Here's how the part is built. I have some questions about the finished solid (model axes, mm). A direction names the side the tool comes from. Round coordinates to 2 decimals unless told otherwise and drop trailing zeros. Loops run counter-clockwise (first coordinate to the right, second up) from the corner with the lowest first, then second, coordinate; pieces in that order, holes last. Notation, with made-up numbers: (-4.75, 68) -> (51.25, 68) arc R21 ccw to (51.25, 76) -> close; hole circle Ø4 at (8, -37). An arc over 180 degrees is marked (long way). Use CSV: the item, a comma, the result in double quotes. Start each with the question number.
from build123d import *

# Parameters (mm, degrees)
F1_DEPTH = 910
F3_DEPTH = 125.001
F5_DEPTH = 65.001
F6_R     = 9
F7_DEPTH = 7.5
F8_R     = 9
F9_DEPTH = 7.5


with BuildPart() as f1:
    # F0 (on Front) → F1 (new body)
    with BuildSketch(Plane.XZ):
        with BuildLine():
            Line((0, 125), (0, 0))
            Line((0, 0), (65, 0))
            Line((65, 0), (65, 7.5))
            Line((65, 7.5), (12.7, 7.5))
            ThreePointArc((12.7, 7.5), (7.043146, 9.843146), (4.7, 15.5))
            Line((4.7, 15.5), (4.7, 109.5))
            ThreePointArc((4.7, 109.5), (7.043146, 115.156854), (12.7, 117.5))
            Line((12.7, 117.5), (65, 117.5))
            Line((65, 117.5), (65, 125))
            Line((65, 125), (0, 125))
        make_face()
    extrude(amount=F1_DEPTH)

    # F2 (on face) → F3 (cut, through all)
    with BuildSketch(Plane.XY.offset(125)):
        Polygon((65, -65), (65, 0), (0, 0), align=None)
    extrude(amount=-F3_DEPTH, mode=Mode.SUBTRACT)

    # F4 (on face) → F5 (cut, through all)
    with BuildSketch(Plane(origin=(0, 0, 0), x_dir=(0, -1, 0), z_dir=(-1, 0, 0))):
        Polygon((910, 0), (910, 125), (785, 125), align=None)
    extrude(amount=-F5_DEPTH, mode=Mode.SUBTRACT)

    # F6 (on face) → F7 (cut, through all)
    with BuildSketch(Plane.XY.offset(125)):
        with Locations((32.5, -350)):
            Circle(F6_R)
        with Locations((32.5, -452)):
            Circle(F6_R)
    extrude(amount=-F7_DEPTH, mode=Mode.SUBTRACT)

    # F8 (on face) → F9 (cut, through all)
    with BuildSketch(Plane.XY.offset(125)):
        with Locations((32.5, -508)):
            Circle(F8_R)
        with Locations((32.5, -610)):
            Circle(F8_R)
    extrude(amount=-F9_DEPTH, mode=Mode.SUBTRACT)


solid = f1.part
Q1. Will these pins go through, and if not, where does the flat tip stop? pin 1 Ø6 at (y, z) = (-340.5, 46) entering from -X; pin 2 Ø6 at (y, z) = (-410.5, 110) entering from +X; pin 3 Ø12 at (y, z) = (-409.5, 96.5) entering from +X.
Q2. I want a section at A-A, the plane x = 32.5. List the corners of the cut face in (y, z) for me, then the cut area to 3 significant figures.
Q3. I need wall thicknesses on line 1 along Z through (x, y) = (17.5, -515); line 2 along Y through (x, z) = (32, 120); line 3 along Y through (x, z) = (32, 122). Which ranges of each line are inside material? Lowest first, please.
Q4. I want a section at B-B, the plane y = -610. List the corners of the cut face in (x, z) for me, then the cut area to 3 significant figures.
Q5. For faces 4 (the cylindrical face through (30.549, -460.786, 121.302)), 5 (the flat face through (3, -3, 67)), 6 (the flat face through (39, -451, 7.5)), which set-ups out of +Z, -Z, +X, -X, +Y, -Y let a thin tool reach every point of the face, with its end or its side?
Q6. I want a section at D-D, the plane z = 97. List the corners of the cut face in (x, y) for me.
Q7. I want a section at C-C, the plane y = -723. List the corners of the cut face in (x, z) for me, then the cut area to 3 significant figures.
Q8. If we mould it in two halves opening along X, with no side actions, what happens to faces 1 (the cylindrical face through (30.549, -618.786, 121.302)), 2 (the flat face through (4.7, -443, 62)), 3 (the flat face through (0, -449, 63))? For each: pulls with the +X half, pulls with the -X half, needs draft (parallel to the pull), parting line crosses it, or undercut.
Values found:
1,pin 1,"x = 0"
1,pin 2,"x = 5.51"
1,pin 3,"x = 4.7"
2,outline,"(-910, 0) -> (-32.5, 0) -> (-32.5, 7.5) -> (-902.5, 7.5) -> close; (-792.5, 117.5) -> (-619, 117.5) -> (-619, 125) -> (-785, 125) -> close; (-601, 117.5) -> (-517, 117.5) -> (-517, 125) -> (-601, 125) -> close; (-499, 117.5) -> (-461, 117.5) -> (-461, 125) -> (-499, 125) -> close; (-443, 117.5) -> (-359, 117.5) -> (-359, 125) -> (-443, 125) -> close; (-341, 117.5) -> (-32.5, 117.5) -> (-32.5, 125) -> (-341, 125) -> close"
2,area,"11,700 mm2"
3,line 1,"0 to 7.5, 117.5 to 125"
3,line 2,"-790 to -618.99, -601.01 to -516.99, -499.01 to -460.99, -443.01 to -358.99, -341.01 to -32"
3,line 3,"-788 to -618.99, -601.01 to -516.99, -499.01 to -460.99, -443.01 to -358.99, -341.01 to -32"
4,outline,"(0, 0) -> (65, 0) -> (65, 7.5) -> (12.7, 7.5) arc R8 cw to (4.7, 15.5) -> (4.7, 109.5) arc R8 cw to (12.7, 117.5) -> (23.5, 117.5) -> (23.5, 125) -> (0, 125) -> close; (41.5, 117.5) -> (65, 117.5) -> (65, 125) -> (41.5, 125) -> close"
4,area,"1,380 mm2"
5,face 4,"+Z"
5,face 5,"+Z, -Z, +X, +Y"
5,face 6,"+X, +Y, -Y"
6,outline,"(0, -813) -> (4.7, -813) -> (4.7, -4.7) -> (0, 0) -> close"
7,outline,"(0, 0) -> (65, 0) -> (65, 7.5) -> (12.7, 7.5) arc R8 cw to (4.7, 15.5) -> (4.7, 109.5) arc R8 cw to (12.7, 117.5) -> (65, 117.5) -> (65, 125) -> (0, 125) -> close"
7,area,"1,520 mm2"
8,face 1,"undercut"
8,face 2,"pulls with the +X half"
8,face 3,"pulls with the -X half"
